Answer from the drawing. Dimensions are ordinates in mm from the lowest x, y and z of the part. A direction names the side the tool comes from. Give positions to 0.01 mm unless a question says otherwise; leave off trailing zeros. Loops run counter-clockwise (first coordinate to the right, second up) from the corner with the lowest first, then second, coordinate; pieces in that order, holes last. Notation, with made-up numbers: (19, 30) - (34, 30) arc R19 cw to (34, 62) - close; hole circle Ø10 at (84, -31). An arc over 180 degrees is marked (long way). Put each result on its own line as item: value. Start each with the question number.
1. A cutting plane is placed at C-C, the plane y = 30. Determine the outline of the cut face in (x, z), plus the area to 3 significant figures.
2. Consider L1, parallel to Y at x = 17, z = 10.5; L2, parallel to X at y = 56, z = 6.5; L3, parallel to Z at x = 28.5, y = 10. Determine where each line is inside the solid, lowest interval first. Write a range as from..to.
3. A cutting plane is placed at B-B, the plane x = 24.5. Determine the outline of the cut face in (y, z).
4. A cutting plane is placed at D-D, the plane x = 4. Determine the outline of the cut face in (y, z), plus the area to 3 significant figures.
5. Given pin 1 Ø6 at (x, z) = (12, 9.5) entering from -Y; pin 2 Ø1.2 at (x, z) = (35.5, 10) entering from -Y; pin 3 Ø3 at (y, z) = (4.5, 7.5) entering from +X, each flat-ended and moving along its own axis, determine where each tip first touches the part or whether it passes through.
6. A cutting plane is placed at A-A, the plane z = 10.75. Determine the outline of the cut face in (x, y).
7. For the marked faces 1, 2, 3, 4 and 5, determine the directions among +Z, -Z, +X, -X, +Y, -Y from which every point of the face is accessible in a straight line to the end or side of a thin tool.
8. For a pull along Y with two mould halves and no side action, classify the marked faces 6, 7 and 8 as released by +Y, released by -Y, zero draft, split by the parting line, or undercut.
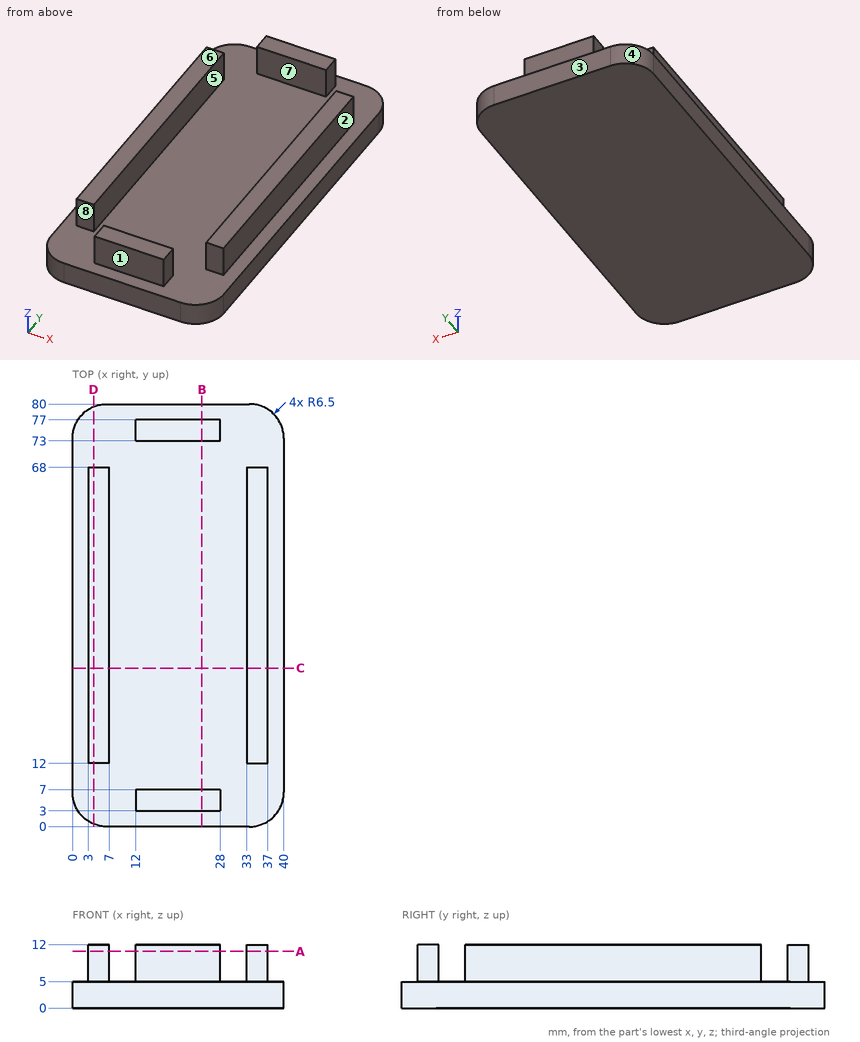
Return value:
1. outline: (0, 0) - (40, 0) - (40, 5) - (37, 5) - (37, 12) - (33, 12) - (33, 5) - (7, 5) - (7, 12) - (3, 12) - (3, 5) - (0, 5) - close
1. area: 256 mm2
2. L1: y = 3..7, 73..77
2. L2: x = 3..7, 33..37
2. L3: z = 0..5
3. outline: (0, 0) - (80, 0) - (80, 5) - (77, 5) - (77, 12) - (73, 12) - (73, 5) - (7, 5) - (7, 12) - (3, 12) - (3, 5) - (0, 5) - close
4. outline: (0.5, 0) - (79.5, 0) - (79.5, 5) - (68, 5) - (68, 12) - (12, 12) - (12, 5) - (0.5, 5) - close
4. area: 787 mm2
5. pin 1: stops at y = 3
5. pin 2: stops at y = 12
5. pin 3: stops at x = 28
6. outline: (3, 12) - (7, 12) - (7, 68) - (3, 68) - close; (12, 3) - (28, 3) - (28, 7) - (12, 7) - close; (12, 73) - (28, 73) - (28, 77) - (12, 77) - close; (33, 12) - (37, 12) - (37, 68) - (33, 68) - close
7. face 1: +Z, +X, -X, -Y
7. face 2: +Z, +X, +Y, -Y
7. face 3: +Z, -Z, +X, -X, +Y
7. face 4: +Z, -Z, -X, +Y
7. face 5: +Z, +Y, -Y
8. face 6: zero draft
8. face 7: undercut
8. face 8: released by -Y
